Check sheet for the drawn part. Datum: minimum x, y, z corner. Units: mm. A direction names the side the tool comes from. Coordinates: 2 decimals unless noted, no trailing zeros. Write each loop counter-clockwise with the first axis right and the second up, starting at its lowest first coordinate (ties: lowest second). Pieces come first, ordered by that corner, then holes. Notation, with made-up numbers: (37.5, 73.5) -> (65.5, 73.5) arc R17 ccw to (65.5, 83.5) -> close; hole circle Ø7 at (52.5, -10). An arc over 180 degrees is marked (long way). Answer in a Markdown table with one row per item. Add a question column.
1. Mould release check, pull along X, two halves, no side actions. Record for the marked faces 3, 4 and 5: pulls with the +X half, pulls with the -X half, needs draft (parallel to the pull), parting line crosses it, or undercut.
2. Set-up check for the marked faces 1 and 2: record each of +Z, -Z, +X, -X, +Y, -Y from which the full face is reachable in a straight line by a thin tool's end or side.
3. Cross-section at D-D on z = 5. Record the cut outline in (x, y).
4. Cross-section at B-B on x = 11. Record the cut outline in (y, z), and give its area (3 significant figures).
5. Depth check by flat-ended pin: P1, Ø1.5, axis at x = 9, y = 20, coming from the -Z side; P2, Ø6, axis at x = 2.5, y = 5.5, coming from the -Z side; P3, Ø1.5, axis at y = 11.5, z = 5, coming from the +X side. Enter the tip coordinate at first touch or a pass-through.
6. Cross-section at C-C on y = 11.75. Record the cut outline in (x, z), and give its area (3 significant figures).
7. Cross-section at A-A on z = 11. Record the cut outline in (x, y).
8. Scan lines: L1, parallel to Z at x = 11, y = 9.75; L2, parallel to Y at x = 2.25, z = 17; L3, parallel to Z at x = 7, y = 2.25. Record each from-to range of solid material in increasing order. Write a range as from..to.
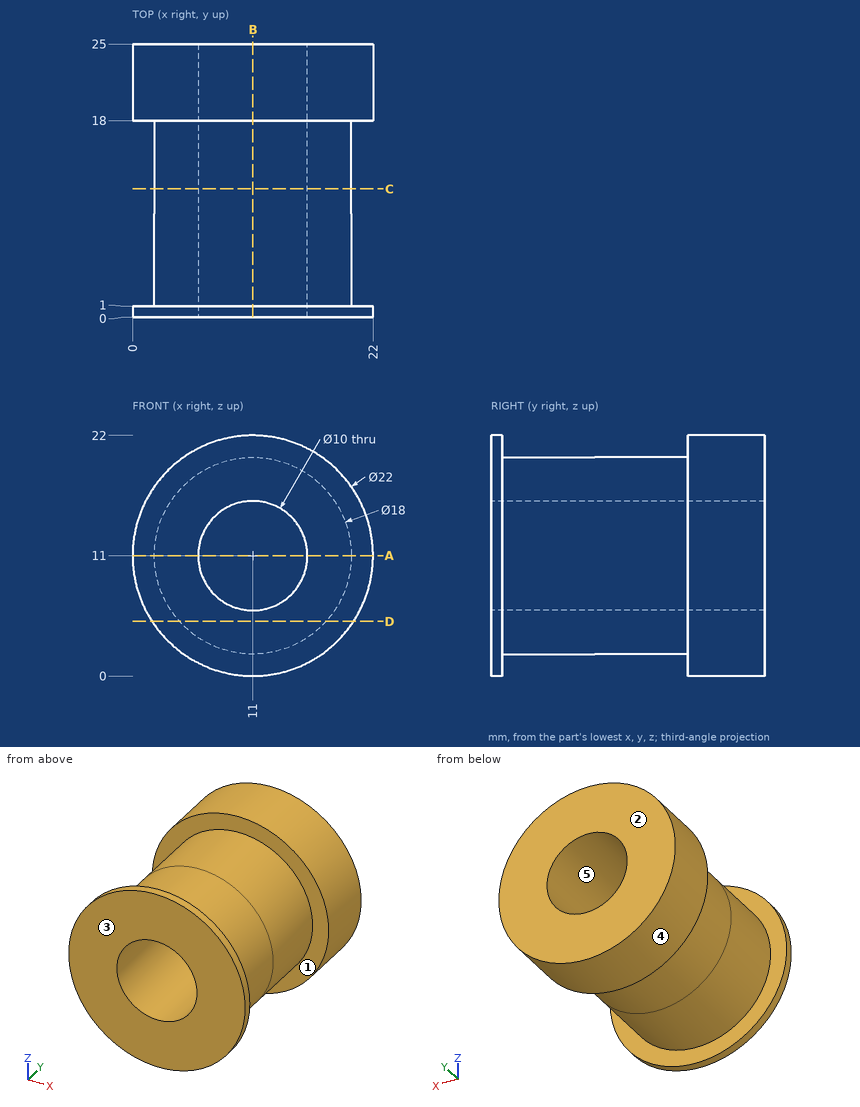
Results found:
| question | item | result |
|---|---|---|
| 1 | face 3 | needs draft |
| 1 | face 4 | parting line crosses it |
| 1 | face 5 | undercut |
| 2 | face 1 | none |
| 2 | face 2 | +Z, -Z, +X, -X, +Y |
| 3 | outline | (1.78, 0) -> (20.22, 0) -> (20.22, 1) -> (17.71, 1) -> (17.71, 18) -> (20.22, 18) -> (20.22, 25) -> (1.78, 25) -> (1.78, 18) -> (4.29, 18) -> (4.29, 1) -> (1.78, 1) -> close |
| 4 | outline | (0, 0) -> (1, 0) -> (1, 2) -> (18, 2) -> (18, 0) -> (25, 0) -> (25, 6) -> (0, 6) -> close; (0, 16) -> (25, 16) -> (25, 22) -> (18, 22) -> (18, 20) -> (1, 20) -> (1, 22) -> (0, 22) -> close |
| 4 | area | 232 mm^2 |
| 5 | P1 | stops at z = 0.07 |
| 5 | P2 | stops at z = 3.88 |
| 5 | P3 | stops at x = 18.31 |
| 6 | outline | circle Ø18 at (11, 11); hole circle Ø10 at (11, 11) |
| 6 | area | 176 mm^2 |
| 7 | outline | (0, 0) -> (6, 0) -> (6, 25) -> (0, 25) -> (0, 18) -> (2, 18) -> (2, 1) -> (0, 1) -> close; (16, 0) -> (22, 0) -> (22, 1) -> (20, 1) -> (20, 18) -> (22, 18) -> (22, 25) -> (16, 25) -> close |
| 8 | L1 | z = 2..6, 16..20 |
| 8 | L2 | y = 0..1, 18..25 |
| 8 | L3 | z = 2.94..8, 14..19.06 |
